Source: three-view drawing plus pictorial views. Frame: mm from the lowest corner of the part. Round coordinates to 2 decimals unless told otherwise and drop trailing zeros. Order: outer loops, then holes, each group sorted by start corner. A loop starts at its lowest first (then second) coordinate and runs counter-clockwise, first axis right, second up. Notation, with made-up numbers: M 71,79 L 77,79 A11 ccw 77,91 Z; hole C 27.25,-22 d6. An arc over 180 degrees is marked long. Return JSON: item names as keys, results as strings. Group by question number.
Q1. Ray query, probe 1 along Z at (x, y) = (18, 2.65) (1 decimal); probe 2 along Z at (x, y) = (28, 1.4); probe 3 along Y at (x, z) = (24, 9.75) (1 decimal). Return the intervals inside material, ascending.
Q2. Cut plane A-A on z = 9.5. Output: boundary loops of the cut face in (x, y).
Q3. Cut plane B-B on y = 0.7. Output: boundary loops of the cut face in (x, z) (1 decimal).
Q4. Cut plane D-D on z = 6.25. Output: boundary loops of the cut face in (x, y).
Q5. Cut plane C-C on x = 32. Output: boundary loops of the cut face in (y, z), and give its area (3 significant figures).
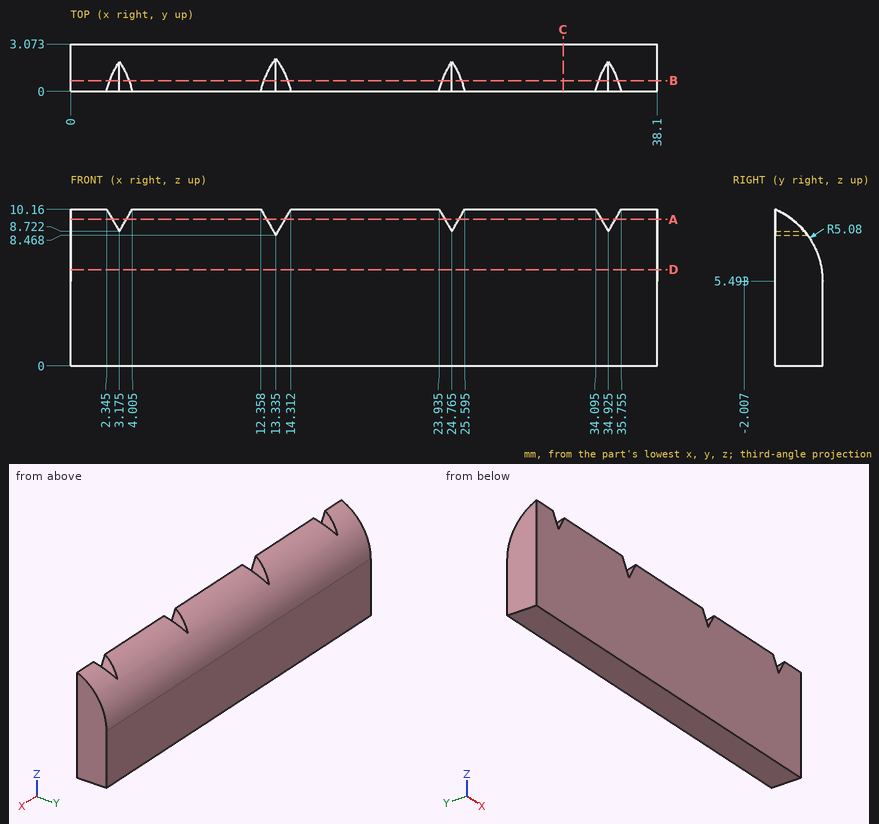
Result sheet:
{
 "1": {"probe 1": "z = 0 to 7.5", "probe 2": "z = 0 to 9.26", "probe 3": "y = 0 to 0.8"},
 "2": {"outline": "M 0,0 L 2.73,0 L 2.73,1.12 L 0,1.12 Z; M 3.62,0 L 12.74,0 L 12.74,1.12 L 3.62,1.12 Z; M 13.93,0 L 24.32,0 L 24.32,1.12 L 13.93,1.12 Z; M 25.21,0 L 34.48,0 L 34.48,1.12 L 25.21,1.12 Z; M 35.37,0 L 38.1,0 L 38.1,1.12 L 35.37,1.12 Z"},
 "3": {"outline": "M 0,0 L 38.1,0 L 38.1,9.8 L 35.5,9.8 L 34.9,8.7 L 34.3,9.8 L 25.4,9.8 L 24.8,8.7 L 24.1,9.8 L 14.1,9.8 L 13.3,8.5 L 12.6,9.8 L 3.8,9.8 L 3.2,8.7 L 2.6,9.8 L 0,9.8 Z"},
 "4": {"outline": "M 0,0 L 38.1,0 L 38.1,3.02 L 0,3.02 Z"},
 "5": {"outline": "M 0,0 L 3.07,0 L 3.07,5.49 A5.08 ccw 0,10.16 Z", "area": "27.2 mm²"}
}
